Autodesk Inventor part; units mm, degrees
ref_plane "YZ Plane" through (0, 0, 0) normal (1, 0, 0) x (0, 1, 0)
ref_plane "XZ Plane" through (0, 0, 0) normal (0, 1, 0) x (-1, 0, 0)
ref_plane "XY Plane" through (0, 0, 0) normal (0, 0, 1) x (1, 0, 0)
sketch "Sketch1" plane through (0, 0, 0) normal (0, 0, 1) x (1, 0, 0)
  line L0 (0, 0) -> (38.8112, 0)
  line L1 (38.8112, 0) -> (38.8112, 19.812)
  line L2 (38.8112, 19.812) -> (0, 19.812)
  line L3 (0, 19.812) -> (0, 0)
  line L4 (-12.7, -12.7) -> (-12.7, 32.512)
  line L5 (-12.7, 32.512) -> (57.8612, 32.512)
  line L6 (57.8612, 32.512) -> (57.8612, -12.7)
  line L7 (-12.7, -12.7) -> (57.8612, -12.7)
  dimension "d0" = 38.8112
  dimension "d1" = 19.812
  dimension "d56" = 12.7
  dimension "d57" = 19.05
extrude "Extrusion1" add sketch "Sketch1" along normal blind 3.175
sketch "Sketch2" plane through (0, 0, 3.175) normal (0, 0, 1) x (1, 0, 0)
  line L0 (0, 19.812) -> (0, 0)
  circle A0 centre (-4.5974, 4.9022) radius 1.0541
  line L1 (38.8112, 19.812) -> (38.8112, 0)
  circle A1 centre (44.9072, 4.9022) radius 1.0541
  circle A2 centre (44.9072, 14.9098) radius 1.0541
  circle A3 centre (-4.5974, 14.9098) radius 1.0541
  circle A4 centre (-4.5974, 4.9022) radius 1.7145
  circle A5 centre (-4.5974, 14.9098) radius 1.7145
  circle A6 centre (44.9072, 14.9098) radius 1.7145
  circle A7 centre (44.9072, 4.9022) radius 1.7145
  dimension "d10" = 2.1082
  dimension "d15" = 3.429
  dimension "d16" = 3.429
  dimension "d17" = 3.429
  dimension "d18" = 3.429
  dimension "d46" = 49.5046
  dimension "d47" = 49.5046
extrude "Extrusion2" cut sketch "Sketch2" against normal blind 3.175 contours A0 | A1 | A2 | A3 | A4 | A5 | A6 | A7
sketch "Sketch3" plane through (57.8612, -12.7, 0) normal (1, 0, 0) x (0, 0, -1)
  line L0 (0, 0) -> (-3.175, 0)
  line L1 (-3.175, 0) -> (-3.175, 45.212)
  line L2 (0, 0) -> (-3.175, 0)
  line L3 (-3.175, 0) -> (-3.175, 45.212)
  line L4 (-3.175, 45.212) -> (0, 45.212)
  line L5 (0, 45.212) -> (0, 0)
  point P0 (0, 12.7)
extrude "Extrusion3" add sketch "Sketch3" along normal blind 3.175
sketch "Sketch4" plane through (0, 0, 3.175) normal (0, 0, 1) x (1, 0, 0)
  line L0 (61.0362, 32.512) -> (61.0362, -12.7)
  line L1 (61.0362, 32.512) -> (57.8612, 32.512)
  line L2 (-12.7, 32.512) -> (61.0362, 32.512)
  line L3 (57.8612, 32.512) -> (51.2299, -12.7)
  line L4 (-12.7, -12.7) -> (61.0362, -12.7)
  line L5 (61.0362, -12.7) -> (51.2299, -12.7)
  point P0 (0, 0)
  dimension "d21" = 3.175
extrude "Extrusion4" add sketch "Sketch4" along normal blind 8.2296
sketch "Sketch8" plane through (0, 0, 3.175) normal (0, 0, 1) x (1, 0, 0)
  line L0 (51.2299, -12.7) -> (32.1799, -12.7)
  line L1 (-12.7, -12.7) -> (51.2299, -12.7)
  line L2 (38.8112, 0) -> (0, 0)
  line L3 (32.1799, -12.7) -> (32.1799, 32.512)
  line L4 (-12.7, 32.512) -> (57.8612, 32.512)
  line L5 (32.1799, 32.512) -> (57.8612, 32.512)
  line L6 (51.2299, -12.7) -> (57.8612, 32.512)
  line L7 (57.8612, 32.512) -> (51.2299, -12.7)
  dimension "d33" = 19.05
  dimension "d36" = 45.212
extrude "Extrusion7" add sketch "Sketch8" along normal blind 8.2296
sketch "Sketch9" plane through (0, 0, 11.4046) normal (0, 0, 1) x (1, 0, 0)
  line L0 (61.0362, -12.7) -> (61.0362, 32.512)
  line L1 (61.0362, 8.6893) -> (74.4982, 8.6893) construction
  line L2 (-12.7, 32.512) -> (61.0362, 32.512)
  line L3 (41.2242, 32.512) -> (63.8302, 32.512) construction
  circle A0 centre (41.2242, 9.906) radius 3.175
  point P0 (0, 0)
  dimension "d41" = 6.35
sketch "Sketch10" plane through (0, 0, 3.175) normal (0, 0, -1) x (-1, 0, 0)
  line L0 (-38.8112, 0) -> (-38.8112, 19.812)
  line L1 (-38.8112, 19.812) -> (-38.8112, 0)
  line L2 (-38.8112, 0) -> (-32.1799, 0)
  line L3 (-32.1799, 32.512) -> (-32.1799, -12.7)
  line L4 (-32.1799, 19.812) -> (-32.1799, 0)
  line L5 (-38.8112, 19.812) -> (0, 19.812)
  line L6 (-38.8112, 19.812) -> (-32.1799, 19.812)
  point P0 (0, 0)
extrude "Extrusion9" cut sketch "Sketch10" against normal blind 5.08
thread "Thread1"
thread "Thread2"
thread "Thread3"
thread "Thread4"
sketch "Sketch11" plane through (0, 0, 11.4046) normal (0, 0, 1) x (1, 0, 0)
  line L0 (32.1799, 32.512) -> (32.1799, -12.7)
  line L1 (32.1799, -12.7) -> (61.0362, -12.7)
  line L2 (61.0362, -12.7) -> (61.0362, 32.512)
  line L3 (61.0362, 32.512) -> (32.1799, 32.512)
  line L4 (32.1799, 32.512) -> (32.1799, -12.7)
  point P0 (0, 0)
extrude "Extrusion10" add sketch "Sketch11" along normal blind 3.2004
sketch "Sketch12" plane through (0, 0, 14.605) normal (0, 0, 1) x (1, 0, 0)
  point P0 (0, 0)
sketch "Sketch13" plane through (0, 0, 14.605) normal (0, 0, 1) x (1, 0, 0)
  line L0 (32.1799, 32.512) -> (32.1799, -12.7)
  line L1 (32.1799, 9.906) -> (41.2223, 9.906)
  line L2 (32.1799, -12.7) -> (61.0362, -12.7)
  line L3 (41.2223, -12.7) -> (41.2223, 9.906)
  circle A0 centre (41.2223, 9.906) radius 3.175
  point P0 (0, 0)
  dimension "d60" = 9.0424
  dimension "d61" = 22.606
  dimension "d62" = 6.35
hole "Hole1" at (41.2223, 9.906, 14.605) direction (0, 0, -1) diameter 6.35 depth 6.35
sketch "Sketch14" plane through (0, 0, 8.255) normal (0, 0, -1) x (-1, 0, 0)
  line L0 (-32.1799, 0) -> (-38.8112, 0)
  line L1 (-32.1799, 0) -> (-38.8112, 0)
  line L2 (-38.8112, 0) -> (-38.8112, 19.812)
  line L3 (-38.8112, 19.812) -> (-32.1799, 19.812)
  line L4 (-32.1799, 19.812) -> (-32.1799, 0)
  point P0 (0, 0)
extrude "Extrusion11" add sketch "Sketch14" along normal blind 0.254
thread "Thread5"
properties part number "ClawServoHolder"
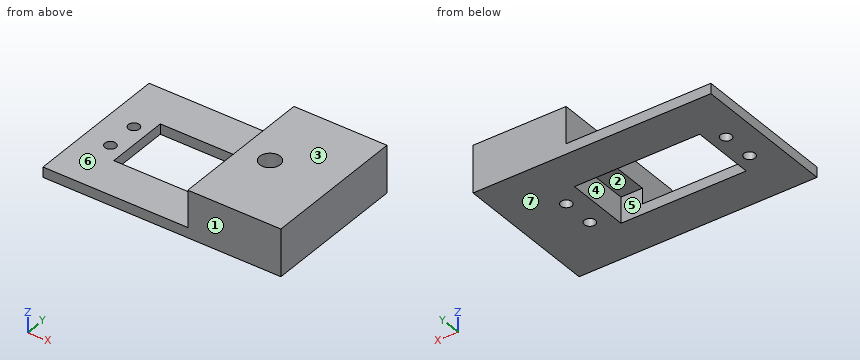
Verification items for the finished model (mm, model axes). Face numbers are marked on the shaded views. A direction names the side the tool comes from. Give positions to 0.01 mm unless a question says otherwise; leave off trailing zeros. Loops run counter-clockwise (first coordinate to the right, second up) from the corner with the lowest first, then second, coordinate; pieces in that order, holes last.
1. Go/stop test with flat-tipped pins: P1, Ø3, axis at y = 8.5, z = 13, coming from the -X side; P2, Ø6, axis at x = 8.5, y = 19, coming from the +Z side (3 decimals); P3, Ø1, axis at x = 45, y = 4.5, coming from the -Z side (3 decimals); P4, Ø5, axis at x = 11.5, z = 7.5, coming from the -Y side. Record where each tip stops, or that it passes through.
Derived:
P1: stops at x = 32.18
P2: stops at z = 3.175
P3: stops at z = 3.175
P4: passes through
2. Cross-section at B-B on z = 6.75. Record the cut outline in (x, y).
Derived:
outline: (32.18, -12.7) - (61.04, -12.7) - (61.04, 32.51) - (32.18, 32.51) - (32.18, 19.81) - (38.81, 19.81) - (38.81, 0) - (32.18, 0) - close
3. Cross-section at A-A on x = 9. Record the cut outline in (y, z) (3 decimals), and give its area (3 significant figures).
Derived:
outline: (-12.7, 0) - (0, 0) - (0, 3.175) - (-12.7, 3.175) - close; (19.812, 0) - (32.512, 0) - (32.512, 3.175) - (19.812, 3.175) - close
area: 80.6 mm2
4. Cross-section at C-C on y = -4. Record the cut outline in (x, z) (3 decimals), and give its area (3 significant figures).
Derived:
outline: (-12.7, 0) - (61.036, 0) - (61.036, 14.605) - (32.18, 14.605) - (32.18, 3.175) - (-12.7, 3.175) - close
area: 564 mm2
5. Tool access check on the marked faces 5, 6 and 7. Record the directions out of +Z, -Z, +X, -X, +Y, -Y that give a thin tool (end or side, any length) a straight path to the whole face; none if there is none.
Derived:
face 5: -Z
face 6: +Z, -X, +Y, -Y
face 7: -Z, +X, -X, +Y, -Y
6. Material ranges on probe 1 along Y at (x, z) = (38, 5.25); probe 2 along X at (y, z) = (30, 8); probe 3 along Z at (x, y) = (-6, 10) (3 decimals), recorded low to high.
Derived:
probe 1: y = -12.7 to 0, 19.81 to 32.51
probe 2: x = 32.18 to 61.04
probe 3: z = 0 to 3.175
7. Release check for a two-part mould opening along Y. For the marked faces 1, 2, 3 and 4 record: +Y half, -Y half, draft (parallel to the pull), parting line (faces both ways), or undercut.
Derived:
face 1: -Y half
face 2: undercut
face 3: draft
face 4: undercut
8. Cross-section at D-D on y = 12. Record the cut outline in (x, z) (3 decimals), and give its area (3 significant figures).
Derived:
outline: (-12.7, 0) - (0, 0) - (0, 3.175) - (-12.7, 3.175) - close; (32.18, 8.001) - (38.811, 8.001) - (38.811, 0) - (61.036, 0) - (61.036, 14.605) - (43.609, 14.605) - (43.609, 8.255) - (38.836, 8.255) - (38.836, 14.605) - (32.18, 14.605) - close
area: 378 mm2
